Autodesk Inventor part; units mm, degrees
ref_plane "YZ Plane" through (0, 0, 0) normal (1, 0, 0) x (0, 1, 0)
ref_plane "XZ Plane" through (0, 0, 0) normal (0, 1, 0) x (-1, 0, 0)
ref_plane "XY Plane" through (0, 0, 0) normal (0, 0, 1) x (1, 0, 0)
sketch "Sketch1" plane through (0, 0, 0) normal (0, 0, 1) x (1, 0, 0)
  line L0 (0, 0) -> (35, 0)
  line L1 (35, 0) -> (35, 14.5)
  line L2 (27.5, 22) -> (7.5, 22)
  line L3 (0, 14.5) -> (0, 0)
  arc A0 (7.5, 22) -> (0, 14.5) centre (7.5, 14.5) ccw
  arc A1 (35, 14.5) -> (27.5, 22) centre (27.5, 14.5) ccw
  point P0 (35, 22)
  point P1 (0, 22)
  dimension "d0" = 35
  dimension "d1" = 22
  dimension "d2" = 7.5
extrude "Extrusion1" add sketch "Sketch1" along normal blind 4.5
sketch "Sketch2" plane through (0, 0, 4.5) normal (0, 0, 1) x (1, 0, 0)
  line L0 (9.5807, 3.0793) -> (25.4203, 3.0793)
  line L1 (28.8863, 6.5453) -> (28.8863, 15.4547)
  line L2 (25.4203, 18.9207) -> (9.5807, 18.9207)
  line L3 (6.1147, 15.4547) -> (6.1147, 6.5453)
  arc A0 (9.5807, 18.9207) -> (6.1147, 15.4547) centre (9.5807, 15.4547) ccw
  arc A1 (28.8863, 15.4547) -> (25.4203, 18.9207) centre (25.4203, 15.4547) ccw
  arc A2 (25.4203, 3.0793) -> (28.8863, 6.5453) centre (25.4203, 6.5453) ccw
  arc A3 (6.1147, 6.5453) -> (9.5807, 3.0793) centre (9.5807, 6.5453) ccw
  line L4 (35, 0) -> (35, 14.5)
  line L5 (0, 0) -> (35, 0)
  line L6 (0, 14.5) -> (0, 0)
  line L7 (27.5, 22) -> (7.5, 22)
  point P0 (29, 19)
  point P1 (29, 3)
  point P2 (6, 19)
  dimension "d5" = 23
  dimension "d6" = 16
  dimension "d7" = 3.466
  dimension "d8" = 3.466
  dimension "d9" = 6.1137
  dimension "d10" = 3.0793
  dimension "d49" = 6.1147
  dimension "d50" = 3.0793
extrude "Extrusion2" add sketch "Sketch2" along normal blind 5
sketch "Sketch3" plane through (0, 0, 0) normal (0, 0, -1) x (-1, 0, 0)
  circle A0 centre (-2, 11) radius 1.56
  circle A1 centre (-33, 11) radius 1.56
  line L0 (0, 14.5) -> (0, 0)
  line L1 (0, 0) -> (-35, 0)
  dimension "d13" = 3.12
  dimension "d14" = 3.12
  dimension "d18" = 2
  dimension "d19" = 31
  dimension "d20" = 11
  dimension "d21" = 11
hole "Hole1" at (2, 11, 0) direction (0, 0, 1) diameter 3.12 end through all
hole "Hole2" at (33, 11, 0) direction (0, 0, 1) diameter 3.12 end through all
sketch "Sketch4" plane through (0, 0, 9.5) normal (0, 0, 1) x (1, 0, 0)
  circle A0 centre (17.3863, 11.0793) radius 4
  line L0 (28.8863, 6.5453) -> (28.8863, 15.4547)
  line L1 (9.5807, 3.0793) -> (25.4203, 3.0793)
  point P0 (0, 0)
  dimension "d36" = 8
  dimension "d37" = 11.5
  dimension "d38" = 8
extrude "Extrusion3" cut sketch "Sketch4" against normal blind 5
sketch "Sketch5" plane through (17.3863, 11.0793, 4.5) normal (0, 0, 1) x (1, 0, 0)
  circle A0 centre (0, 0) radius 1.55
  circle A1 centre (0, 0) radius 4
  point P0 (-17.3863, -11.0793)
  dimension "d41" = 3.1
  dimension "d42" = 2.45
extrude "Extrusion4" cut sketch "Sketch5" against normal blind 2.15 contours A0
sketch "Sketch6" plane through (17.3863, 11.0793, 2.35) normal (0, 0, 1) x (1, 0, 0)
  circle A0 centre (0.0058, 0.0144) radius 1.005
  circle A1 centre (0, 0) radius 1.55
  point P0 (-17.3863, -11.0793)
  dimension "d45" = 2.01
  dimension "d46" = 0.5295
extrude "Extrusion5" cut sketch "Sketch6" against normal through all contours A0
properties part number "Aquamote3.2_housing_cap"
Read the model definition and answer for the solid it produces. Units are mm, in the model's axes. A direction names the side the tool comes from. Give positions to 0.01 mm unless a question says otherwise; leave off trailing zeros. Write each loop counter-clockwise with the first axis right and the second up, starting at its lowest first coordinate (ties: lowest second). Pieces come first, ordered by that corner, then holes. Notation, with made-up numbers: (79, 3) -> (123, 3) arc R17 ccw to (123, 23) -> close; hole circle Ø10 at (77.5, 33). An arc over 180 degrees is marked (long way). Answer as a JSON object with one key per item and string values. Group by question number.
1) A tool of negligible diameter and unlimited length cuts with its end or side. For faces 1 (the flat face through (18, 18.921, 7)), 2 (the flat face through (17, 3.079, 7)), 3 (the flat face through (28.886, 11, 7)), 4 (the flat face through (19.1, 11.1, 4.5)), 5 (the cylindrical face through (7.157, 4.068, 6.965)), from which of +Z, -Z, +X, -X, +Y, -Y can it reach the whole face along a straight path? Write none if from no direction.
2) Find section D-D (z = 2). Write down the section's boundary in (x, y) (3 decimals).
3) The mould has two halves that part along Y. Classify faces 6 (the flat face through (0, 7, 2)), 7 (the cylindrical face through (2.139, 19.745, 2.218)), 8 (the cylindrical face through (21.2, 12.28, 7.04)): +Y half, -Y half, draft (parallel to the pull), parting line (faces both ways), or undercut.
4) Find section A-A (x = 2). Write down the section's boundary in (y, z), and give its area (3 significant figures).
5) Find section B-B (z = 6.75). Write down the section's boundary in (x, y).
6) Find section C-C (x = 28.5). Write down the section's boundary in (y, z).
7) Each of these flat-tipped pins is pushed along its axis until it touches: P1, Ø5.5, axis at x = 17.5, z = 8, coming from the +Y side; P2, Ø2.5, axis at y = 10.5, z = 7.5, coming from the +X side; P3, Ø2, axis at x = 7, z = 6, coming from the -Y side; P4, Ø5.5, axis at x = 20, z = 6.5, coming from the -Y side. Where does it stop, or does it pass through?
8) Consider L1, parallel to X at y = 11, z = 2.5; L2, parallel to Y at x = 17.5, z = 3; L3, parallel to Z at x = 4, y = 17. Determine where each line is inside the solid, lowest interval first. Write a range as from..to.
Values follow:
{
 "1": {"face 1": "+Z, +X, -X, +Y", "face 2": "+Z, +X, -X, -Y", "face 3": "+Z, +X, +Y, -Y", "face 4": "+Z", "face 5": "+Z, -X, -Y"},
 "2": {"outline": "(0, 0) -> (35, 0) -> (35, 14.5) arc R7.5 ccw to (27.5, 22) -> (7.5, 22) arc R7.5 ccw to (0, 14.5) -> close; hole circle Ø3.12 at (2, 11); hole circle Ø2.01 at (17.392, 11.094); hole circle Ø3.12 at (33, 11)"},
 "3": {"face 6": "draft", "face 7": "+Y half", "face 8": "undercut"},
 "4": {"outline": "(0, 0) -> (9.44, 0) -> (9.44, 4.5) -> (0, 4.5) -> close; (12.56, 0) -> (19.6, 0) -> (19.6, 4.5) -> (12.56, 4.5) -> close", "area": "74.2 mm2"},
 "5": {"outline": "(6.11, 6.55) arc R3.47 ccw to (9.58, 3.08) -> (25.42, 3.08) arc R3.47 ccw to (28.89, 6.55) -> (28.89, 15.45) arc R3.47 ccw to (25.42, 18.92) -> (9.58, 18.92) arc R3.47 ccw to (6.11, 15.45) -> close; hole circle Ø8 at (17.39, 11.08)"},
 "6": {"outline": "(0, 0) -> (21.93, 0) -> (21.93, 4.5) -> (17.04, 4.5) -> (17.04, 9.5) -> (4.96, 9.5) -> (4.96, 4.5) -> (0, 4.5) -> close"},
 "7": {"P1": "stops at y = 18.92", "P2": "stops at x = 28.89", "P3": "stops at y = 3.46", "P4": "stops at y = 0"},
 "8": {"L1": "x = 0..0.44, 3.56..15.84, 18.93..31.44, 34.56..35", "L2": "y = 0..9.53, 12.63..22", "L3": "z = 0..4.5"}
}
